Geometry check sheet. Reference: the model listing, model coordinates, mm. Coordinates: 2 decimals unless noted, no trailing zeros. Order: outer loops, then holes, each group sorted by start corner. A loop starts at its lowest first (then second) coordinate and runs counter-clockwise, first axis right, second up. Notation, with made-up numbers: (15, -35.5) -> (43, -35.5) arc R8 cw to (43, -24.5) -> close; hole circle Ø7 at (41, -39). An arc over 180 degrees is marked (long way). Answer in a Markdown table with one row per item. Add a question column.
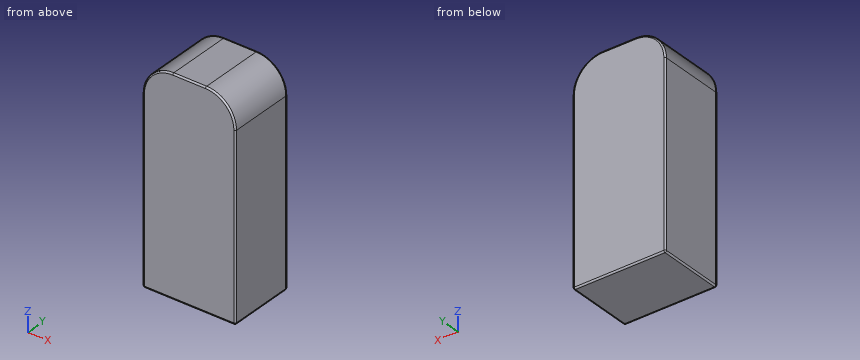
```python
from build123d import *

# Parameters (mm, degrees)
SKETCH1_W           = 62
SKETCH1_H           = 45
BOSS_EXTRUDE1_DEPTH = 142
FILLET1_R           = 20
FILLET2_R           = 1


with BuildPart() as part:
    # Sketch1 → Boss-Extrude1 (new body)
    with BuildSketch(Plane.XY):
        Rectangle(SKETCH1_W, SKETCH1_H)
    extrude(amount=BOSS_EXTRUDE1_DEPTH)

    # Fillet1
    fillet1_edges = [part.edges().sort_by_distance(p)[0] for p in [
        (31, 0, 142),
        (-31, 0, 142),
    ]]
    fillet(fillet1_edges, radius=FILLET1_R)

    # Fillet2
    fillet2_edges = [part.edges().sort_by_distance(p)[0] for p in [
        (0, -22.5, 142),
        (0, 22.5, 142),
        (31, -22.5, 61),
        (-31, -22.5, 61),
        (25.142135624, -22.5, 136.142135624),
        (-25.142135624, -22.5, 136.142135624),
        (-31, 22.5, 61),
        (31, 22.5, 61),
        (25.142135624, 22.5, 136.142135624),
        (-25.142135624, 22.5, 136.142135624),
        (0, 22.5, 0),
        (31, 0, 0),
        (0, -22.5, 0),
        (-31, 0, 0),
    ]]
    fillet(fillet2_edges, radius=FILLET2_R)


solid = part.part
```
(1) Go/stop test with a flat-tipped pin: P1, Ø8, axis at x = 24.5, y = -15.5, coming from the +Z side. Record where the tip stops, or that it passes through.
(2) Scan lines: line 1 along X through (y, z) = (18.5, 122.5); line 2 along Z through (x, y) = (20.5, -8); line 3 along X through (y, z) = (-9.5, 135). Record each from-to range of solid material in increasing order.
(3) Cross-section at A-A (y = 9). Enter the section's corners in (x, z).
Checks:
| question | item | result |
|---|---|---|
| 1 | P1 | z = 139.6 |
| 2 | line 1 | -30.99 to 30.99 |
| 2 | line 2 | 0 to 139.6 |
| 2 | line 3 | -26.2 to 26.2 |
| 3 | outline | (-31, 1) arc R1 ccw to (-30, 0) -> (30, 0) arc R1 ccw to (31, 1) -> (31, 122) arc R20 ccw to (11, 142) -> (-11, 142) arc R20 ccw to (-31, 122) -> close |
